from build123d import *

# Parameters (mm, degrees)
F1_DEPTH = 13
F2_R     = 5


with BuildPart() as f1:
    # F0 (on Top) → F1 (new body)
    with BuildSketch(Plane.XY):
        Polygon((-62.404933, 2.5), (-62.404933, 0), (37.595067, 0), (37.595067, -35), (40.095067, -35), (40.095067, 27.5), (37.595067, 27.5), (37.595067, 2.5), align=None)
    extrude(amount=-F1_DEPTH)

    # F2
    f2_edges = [f1.edges().sort_by_distance(p)[0] for p in [
        (37.595067, 0, -6.5),
        (37.595067, 2.5, -6.5),
    ]]
    fillet(f2_edges, radius=F2_R)


solid = f1.part
Build history of the part. All positions in model axes, mm. A direction names the side the tool comes from. Give positions to 0.01 mm unless a question says otherwise; leave off trailing zeros. Order: outer loops, then holes, each group sorted by start corner. A loop starts at its lowest first (then second) coordinate and runs counter-clockwise, first axis right, second up. Notation, with made-up numbers: M -8,34.5 L 31,34.5 A19 cw 31,52.5 Z; hole C -7.75,-26.75 d11. An arc over 180 degrees is marked long. Put each result on its own line as item: value.
Item 1: Slice it at B-B, the plane x = -48. Write the cut outline in (y, z).
From the geometry:
outline: M 0,-13 L 2.5,-13 L 2.5,0 L 0,0 Z
Item 2: Probe line 1 (Y direction, x = 15, z = -1.5); line 2 (X direction, y = -26, z = -0.5); line 3 (X direction, y = -4, z = -3.75). List the from-to ranges inside material, lowest first. Write a range as [from, to].
From the geometry:
line 1: y = [0, 2.5]
line 2: x = [37.6, 40.1]
line 3: x = [37.49, 40.1]
Item 3: 3-axis set-ups, long thin cutter, end or side, ignore diameter. For faces 1 (the flat face through (37.595, 18, -6)), 2 (the flat face through (-62.405, 1, -6)), 3 (the flat face through (37.595, -20, -6)): which of +Z, -Z, +X, -X, +Y, -Y reach the whole face in a straight line?
From the geometry:
face 1: +Z, -Z, -X, +Y
face 2: +Z, -Z, -X, +Y, -Y
face 3: +Z, -Z, -X, -Y
Item 4: Flat gauge pins, fed straight in: pin 1 Ø1 at (x, z) = (-3.5, -3) entering from -Y; pin 2 Ø6.5 at (y, z) = (-22, -8) entering from -X. Where does each tip first touch, or does it go through?
From the geometry:
pin 1: stops at y = 0
pin 2: stops at x = 37.6
Item 5: Slice it at C-C, the plane y = 16.5. Write the cut outline in (x, z), plus the area to 3 significant figures.
From the geometry:
outline: M 37.6,-13 L 40.1,-13 L 40.1,0 L 37.6,0 Z
area: 32.5 mm2
Item 6: Slice it at A-A, the plane z = -3.5. Write the cut outline in (x, y), plus the area to 3 significant figures.
From the geometry:
outline: M -62.4,0 L 32.6,0 A5 cw 37.6,-5 L 37.6,-35 L 40.1,-35 L 40.1,27.5 L 37.6,27.5 L 37.6,7.5 A5 cw 32.6,2.5 L -62.4,2.5 Z
area: 417 mm2
